from build123d import *

# Parameters (mm, degrees)
SALIENTE_EXTRUIR1_DEPTH = 40
CORTAR_EXTRUIR1_DEPTH   = 40
CROQUIS3_R              = 4
CORTAR_EXTRUIR2_DEPTH   = 40
CORTAR_EXTRUIR3_DEPTH   = 40
CROQUIS5_W              = 5
CROQUIS5_H              = 19
CORTAR_EXTRUIR4_DEPTH   = 40


with BuildPart() as part:
    # Croquis1 → Saliente-Extruir1 (new body)
    with BuildSketch(Plane.XY):
        Polygon((0, 0), (-20, 0), (-20, 20), (-19, 20), (-19, 1), (-1, 1), (-1, 20), (0, 20), align=None)
    extrude(amount=-SALIENTE_EXTRUIR1_DEPTH)

    # Croquis2 → Cortar-Extruir1 (cut)
    with BuildSketch(Plane(origin=(0, 0, 0), x_dir=(0, 0, -1), z_dir=(1, 0, 0))):
        with BuildLine():
            ThreePointArc((30, 20), (37.071067812, 17.071067812), (40, 10))
            Line((40, 10), (40, 20))
            Line((40, 20), (30, 20))
        make_face()
        with BuildLine():
            Line((40, 0), (40, 10))
            ThreePointArc((40, 10), (37.071067812, 2.928932188), (30, 0))
            Line((30, 0), (40, 0))
        make_face()
    extrude(amount=-CORTAR_EXTRUIR1_DEPTH, mode=Mode.SUBTRACT)

    # Croquis3 → Cortar-Extruir2 (cut)
    with BuildSketch(Plane(origin=(0, 0, 0), x_dir=(0, 0, -1), z_dir=(1, 0, 0))):
        with Locations((33.7, 10)):
            Circle(CROQUIS3_R)
    extrude(amount=-CORTAR_EXTRUIR2_DEPTH, mode=Mode.SUBTRACT)

    # Croquis4 → Cortar-Extruir3 (cut)
    with BuildSketch(Plane(origin=(0, 0, 0), x_dir=(-1, 0, 0), z_dir=(0, -1, 0))):
        Polygon((19, 26), (1, 26), (1, 34.358898944), (9.832157659, 34.358898944), (19, 34.358898944), align=None)
    extrude(amount=-CORTAR_EXTRUIR3_DEPTH, mode=Mode.SUBTRACT)

    # Croquis5 → Cortar-Extruir4 (cut)
    with BuildSketch(Plane.XZ):
        with Locations((-10, -12.5)):
            Rectangle(CROQUIS5_W, CROQUIS5_H)
    extrude(amount=-CORTAR_EXTRUIR4_DEPTH, mode=Mode.SUBTRACT)


solid = part.part
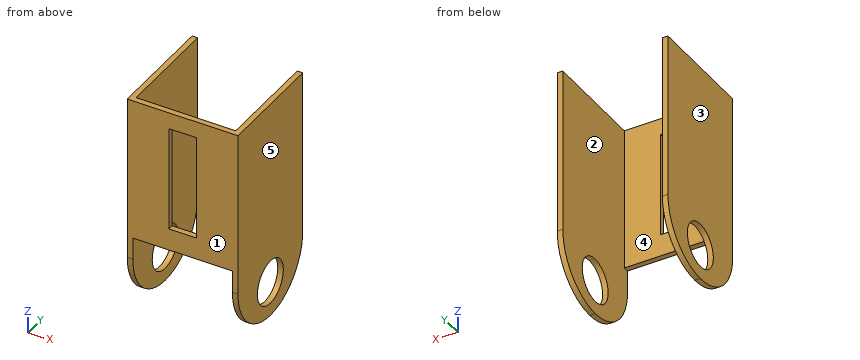
Geometry: final body of the model. Coordinates: model frame, mm. Face numbers are marked on the shaded views. A direction names the side the tool comes from. Coordinates: 2 decimals unless noted, no trailing zeros. Order: outer loops, then holes, each group sorted by start corner. A loop starts at its lowest first (then second) coordinate and runs counter-clockwise, first axis right, second up.
(1) Material intervals for probe 1 along X at (y, z) = (9.5, -3); probe 2 along Z at (x, y) = (-19.7, 10); probe 3 along Y at (x, z) = (-15, -18.5), sorted ascending.
(2) Draft query along X for the marked faces 1, 2 and 3. Return one class per face: pulls with the +X half, pulls with the -X half, needs draft (parallel to the pull), parting line crosses it, or undercut.
(3) First-contact query: pin 1 (5.5 mm diameter, centred on x = -11.5, z = -15, fed in from +Y); pin 2 (1.1 mm diameter, centred on x = -6.5, y = 0.5, fed in from -Z). Flat tips, straight axial feed; report the tip coordinate or a pass-through.
(4) Section query B-B (z = -16.5). Return the cut outline in (x, y), plus the area to 3 significant figures.
(5) Section query A-A (x = -10.25). Return the cut outline in (y, z), plus the area to 3 significant figures.
(6) Section query D-D (y = 12.75). Return the cut outline in (x, z).
(7) Section query C-C (z = -33.7). Return the cut outline in (x, y).
(8) Access query for the marked faces 4 and 5. Directions: +Z, -Z, +X, -X, +Y, -Y. A direction counts if a zero-diameter tool reaches every point of the face in a straight line with its end or side. Return the directions, or none.
Solution:
1. probe 1: x = -20 to -19, -1 to 0
1. probe 2: z = -40 to -37.7, -29.7 to 0
1. probe 3: y = 0 to 1
2. face 1: needs draft
2. face 2: undercut
2. face 3: pulls with the -X half
3. pin 1: stops at y = 1
3. pin 2: stops at z = -26
4. outline: (-20, 0) - (-12.5, 0) - (-12.5, 1) - (-19, 1) - (-19, 20) - (-20, 20) - close; (-7.5, 0) - (0, 0) - (0, 20) - (-1, 20) - (-1, 1) - (-7.5, 1) - close
4. area: 53.0 mm2
5. outline: (0, -26) - (1, -26) - (1, -22) - (0, -22) - close; (0, -3) - (1, -3) - (1, 0) - (0, 0) - close
5. area: 7.00 mm2
6. outline: (-20, -39.61) - (-19, -39.61) - (-19, -36.6) - (-20, -36.6) - close; (-20, -30.8) - (-19, -30.8) - (-19, 0) - (-20, 0) - close; (-1, -39.61) - (0, -39.61) - (0, -36.6) - (-1, -36.6) - close; (-1, -30.8) - (0, -30.8) - (0, 0) - (-1, 0) - close
7. outline: (-20, 0.71) - (-19, 0.71) - (-19, 6) - (-20, 6) - close; (-20, 14) - (-19, 14) - (-19, 19.29) - (-20, 19.29) - close; (-1, 0.71) - (0, 0.71) - (0, 6) - (-1, 6) - close; (-1, 14) - (0, 14) - (0, 19.29) - (-1, 19.29) - close
8. face 4: +Z, -Z, +Y
8. face 5: +Z, -Z, +X, +Y, -Y
